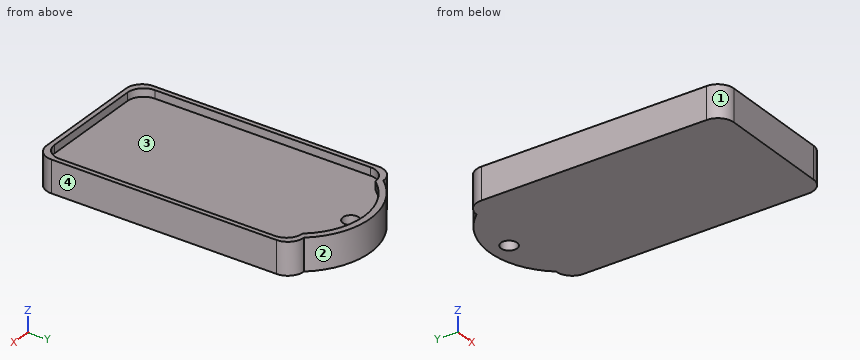
from build123d import *

# Parameters (mm, degrees)
F1_DEPTH = 10
F2_R     = 2.5
F3_DEPTH = 2.5
F4_DEPTH = 40.9


with BuildPart() as f1:
    # F0 (on Top) → F1 (new body)
    with BuildSketch(Plane.XY):
        with BuildLine():
            ThreePointArc((33.0953783914, 67.4970372766), (15.5953783914, 75.7789746896), (-1.9046216086, 67.4970372766))
            Line((-1.9046216086, 67.4970372766), (33.0953783914, 67.4970372766))
        make_face()
        with BuildLine():
            ThreePointArc((-6.9046216086, -7.5029627234), (-5.4401555145, -11.0384966293), (-1.9046216086, -12.5029627234))
            Line((-1.9046216086, -12.5029627234), (33.0953783914, -12.5029627234))
            ThreePointArc((33.0953783914, -12.5029627234), (36.6309122974, -11.0384966293), (38.0953783914, -7.5029627234))
            Line((38.0953783914, -7.5029627234), (38.0953783914, 62.4970372766))
            ThreePointArc((38.0953783914, 62.4970372766), (36.6309122974, 66.0325711826), (33.0953783914, 67.4970372766))
            Line((33.0953783914, 67.4970372766), (-1.9046216086, 67.4970372766))
            ThreePointArc((-1.9046216086, 67.4970372766), (-5.4401555145, 66.0325711826), (-6.9046216086, 62.4970372766))
            Line((-6.9046216086, 62.4970372766), (-6.9046216086, -7.5029627234))
        make_face()
    extrude(amount=F1_DEPTH)

    # F2 (on face) → F3 (cut)
    with BuildSketch(Plane.XY.offset(10)):
        with BuildLine():
            ThreePointArc((31.6309122974, 66.0325711826), (15.5953783914, 73.7975858827), (-0.4401555145, 66.0325711826))
            Line((-0.4401555145, 66.0325711826), (31.6309122974, 66.0325711826))
        make_face()
        with Locations((15.5847426504, 69.739215076)):
            Circle(F2_R, mode=Mode.SUBTRACT)
        with BuildLine():
            ThreePointArc((-5.4401555145, -6.0384966293), (-3.9756894204, -9.5740305352), (-0.4401555145, -11.0384966293))
            Line((-0.4401555145, -11.0384966293), (31.6309122974, -11.0384966293))
            ThreePointArc((31.6309122974, -11.0384966293), (35.1664462033, -9.5740305352), (36.6309122974, -6.0384966293))
            Line((36.6309122974, -6.0384966293), (36.6309122974, 61.0325711826))
            ThreePointArc((36.6309122974, 61.0325711826), (35.1664462033, 64.5681050885), (31.6309122974, 66.0325711826))
            Line((31.6309122974, 66.0325711826), (-0.4401555145, 66.0325711826))
            ThreePointArc((-0.4401555145, 66.0325711826), (-3.9756894204, 64.5681050885), (-5.4401555145, 61.0325711826))
            Line((-5.4401555145, 61.0325711826), (-5.4401555145, -6.0384966293))
        make_face()
    extrude(amount=-F3_DEPTH, mode=Mode.SUBTRACT)

    # F4 (cut): a face of the model
    f4_faces = [f1.faces().sort_by_distance(p)[0] for p in [
        (15.5847426504, 69.739215076, 10),
    ]]
    extrude(f4_faces, amount=-F4_DEPTH, mode=Mode.SUBTRACT)


solid = f1.part
Can you work these out from the model? Positions are in its coordinate system, mm. Face numbers are marked on the shaded views. Give positions to 0.01 mm unless a question says otherwise; leave off trailing zeros. Order: outer loops, then holes, each group sorted by start corner. A loop starts at its lowest first (then second) coordinate and runs counter-clockwise, first axis right, second up. Notation, with made-up numbers: M -24.5,50 L -2.5,50 A16 cw -2.5,75 Z; hole C 31,-32 d1. An arc over 180 degrees is marked long. Use a Markdown table: item, result. Add a question column.
Item 1: Suppose I cut it at A-A (z = 8.5). List the corners of the cut face in (x, y) for me.
Item 2: We'd pull the mould along Y, two halves only. Please class the marked faces 1, 2, 3 and 4: +Y half, -Y half, draft (parallel to the pull), parting line (faces both ways), or undercut.
Item 3: Suppose I cut it at C-C (x = 1). List the corners of the cut face in (y, z) for me.
Item 4: Suppose I cut it at D-D (z = 2.75). List the corners of the cut face in (x, y) for me, then the cut area to 3 significant figures.
Item 5: Will these pins go through, and if not, where does the flat tip stop? pin 1 (12.5 mm diameter, centred on x = 17.5, y = 35.5, fed in from +Z); pin 2 (1.2 mm diameter, centred on x = 17.5, z = 8.5, fed in from +Y).
Item 6: If I drill on L1, parallel to X at y = 47.5, z = 8.25; L2, parallel to Z at x = 22, y = 8.5; L3, parallel to Y at x = 19.5, z = 8.5, over which ranges is the centre line in solid material (lowest first)? Write a range as [from, to].
Item 7: Suppose I cut it at B-B (y = 1). List the corners of the cut face in (x, z) for me, then the cut area to 3 significant figures.
Answer sheet:
| question | item | result |
|---|---|---|
| 1 | outline | M -6.9,-7.5 A5 ccw -1.9,-12.5 L 33.1,-12.5 A5 ccw 38.1,-7.5 L 38.1,62.5 A5 ccw 33.1,67.5 A22.63 ccw -1.9,67.5 A5 ccw -6.9,62.5 Z; hole M -5.44,-6.04 A5 ccw -0.44,-11.04 L 31.63,-11.04 A5 ccw 36.63,-6.04 L 36.63,61.03 A5 ccw 31.63,66.03 A20.44 ccw -0.44,66.03 A5 ccw -5.44,61.03 Z |
| 2 | face 1 | -Y half |
| 2 | face 2 | +Y half |
| 2 | face 3 | undercut |
| 2 | face 4 | draft |
| 3 | outline | M -12.5,0 L 70.44,0 L 70.44,10 L 67.67,10 L 67.67,7.5 L -11.04,7.5 L -11.04,10 L -12.5,10 Z |
| 4 | outline | M -6.9,-7.5 A5 ccw -1.9,-12.5 L 33.1,-12.5 A5 ccw 38.1,-7.5 L 38.1,62.5 A5 ccw 33.1,67.5 A22.63 ccw -1.9,67.5 A5 ccw -6.9,62.5 Z; hole C 15.58,69.74 d5 |
| 4 | area | 3,760 mm² |
| 5 | pin 1 | stops at z = 7.5 |
| 5 | pin 2 | stops at y = 75.74 |
| 6 | L1 | x = [-6.9, -5.44], [36.63, 38.1] |
| 6 | L2 | z = [0, 7.5] |
| 6 | L3 | y = [-12.5, -11.04], [73.42, 75.44] |
| 7 | outline | M -6.9,0 L 38.1,0 L 38.1,10 L 36.63,10 L 36.63,7.5 L -5.44,7.5 L -5.44,10 L -6.9,10 Z |
| 7 | area | 345 mm² |
